Could you check a few things on this model? Use its own coordinates, in mm. Round coordinates to 2 decimals unless told otherwise and drop trailing zeros. Loops run counter-clockwise (first coordinate to the right, second up) from the corner with the lowest first, then second, coordinate; pieces in that order, holes last. Notation, with made-up numbers: M 89.5,19.5 L 146.5,19.5 A12 cw 146.5,39.5 Z; hole C -27,24.5 d6. An arc over 180 degrees is marked long. Answer in a Markdown table with one row per item.
```python
from build123d import *

# Parameters (mm, degrees)
SKETCH1_R           = 1.65
SKETCH1_R_2         = 2.7
BOSS_EXTRUDE1_DEPTH = 6.35


with BuildPart() as part:
    # Sketch1 → Boss-Extrude1 (new body)
    with BuildSketch(Plane(origin=(-388.62, 0, 0), x_dir=(0, -1, 0), z_dir=(-1, 0, 0))):
        Polygon((-371.45, -148.811863322), (-365.1, -148.811863322), (-365.1, -186.911863322), (-328.298226018, -196.772868941), (-329.941726955, -202.906497938), (-305.407210967, -209.480501683), (-303.763710031, -203.346872686), (-194.817257994, -232.538986528), (-196.46075893, -238.672615525), (-171.926242943, -245.24661927), (-170.282742006, -239.112990273), (-61.336289969, -268.305104115), (-62.979790906, -274.438733112), (-38.445274918, -281.012736857), (-36.801773982, -274.87910786), (0, -284.740113479), (0, -3.788281448), (-365.1, -3.788281448), (-365.1, -41.888281448), (-371.45, -41.888281448), (-371.45, -67.288281448), (-365.1, -67.288281448), (-365.1, -123.411863322), (-371.45, -123.411863322), align=None)
        with Locations(Location((-49.890782444, -274.658920486, 0), (0, 0, 90))):
            Circle(SKETCH1_R, mode=Mode.SUBTRACT)
        with Locations(Location((-368.275, -54.588281448, 0), (0, 0, 90))):
            Circle(SKETCH1_R, mode=Mode.SUBTRACT)
        with Locations(Location((-183.371750468, -238.892802899, 0), (0, 0, 90))):
            Circle(SKETCH1_R, mode=Mode.SUBTRACT)
        with Locations(Location((-368.275, -136.111863322, 0), (0, 0, 90))):
            Circle(SKETCH1_R, mode=Mode.SUBTRACT)
        with Locations(Location((-316.852718493, -203.126685312, 0), (0, 0, 90))):
            Circle(SKETCH1_R, mode=Mode.SUBTRACT)
        with Locations(Location((-294.45, -29.188301448, 0), (0, 0, 90))):
            Circle(SKETCH1_R_2, mode=Mode.SUBTRACT)
        with Locations(Location((-207.55, -29.188301448, 0), (0, 0, 90))):
            Circle(SKETCH1_R_2, mode=Mode.SUBTRACT)
        with Locations(Location((-120.65, -29.188301448, 0), (0, 0, 90))):
            Circle(SKETCH1_R_2, mode=Mode.SUBTRACT)
        with Locations(Location((-33.74898, -181.588301448, 0), (0, 0, 90))):
            Circle(SKETCH1_R_2, mode=Mode.SUBTRACT)
        with Locations(Location((-33.74898, -29.188301448, 0), (0, 0, 90))):
            Circle(SKETCH1_R_2, mode=Mode.SUBTRACT)
        with Locations(Location((-33.74898, -130.788301448, 0), (0, 0, 90))):
            Circle(SKETCH1_R_2, mode=Mode.SUBTRACT)
        with Locations(Location((-33.74898, -79.988301448, 0), (0, 0, 90))):
            Circle(SKETCH1_R_2, mode=Mode.SUBTRACT)
    extrude(amount=-BOSS_EXTRUDE1_DEPTH)


solid = part.part
```
1) I want a section at A-A, the plane z = -158. Please give me the cut outline in (x, y), plus the area to 3 significant figures.
Computed:
| item | result |
|---|---|
| outline | M -388.62,0 L -382.27,0 L -382.27,365.1 L -388.62,365.1 Z |
| area | 2,320 mm² |
2) I want a section at B-B, the plane y = 272. Please give me the cut outline in (x, z), plus the area to 3 significant figures.
Computed:
| item | result |
|---|---|
| outline | M -388.62,-211.86 L -382.27,-211.86 L -382.27,-3.79 L -388.62,-3.79 Z |
| area | 1,320 mm² |
3) Will these pins go through, and if not, where does the flat tip stop? P1, Ø3, axis at x = -384, z = -24.5, coming from the +Y side; P2, Ø4.5, axis at y = 33.75, z = -181.59, coming from the +X side; P3, Ø1.9, axis at x = -385.5, y = 367.5, coming from the +Z side; P4, Ø1.9, axis at x = -385, y = 367.5, coming from the -Z side.
Computed:
| item | result |
|---|---|
| P1 | stops at y = 365.1 |
| P2 | passes through |
| P3 | stops at z = -41.89 |
| P4 | stops at z = -148.81 |
4) I need wall thicknesses on line 1 (Y direction, x = -385, z = -29.5); line 2 (Y direction, x = -383, z = -55); line 3 (Y direction, x = -385.5, z = -136). Which ranges of each line are inside material? Lowest first, please.
Computed:
| item | result |
|---|---|
| line 1 | y = 0 to 31.07, 36.43 to 117.97, 123.33 to 204.87, 210.23 to 291.77, 297.13 to 365.1 |
| line 2 | y = 0 to 366.68, 369.87 to 371.45 |
| line 3 | y = 0 to 366.63, 369.92 to 371.45 |
5) If we mould it in two halves opening along Y, with no side actions, what happens to faces 1 (the face through (-382.27, 188, -111)), 2 (the face through (-385.489, 346.957, -191.773)), 3 (the face through (-385.49, 18.66, -279.74))? For each: released by +Y, released by -Y, zero draft, split by the parting line, or undercut.
Computed:
| item | result |
|---|---|
| face 1 | zero draft |
| face 2 | released by +Y |
| face 3 | undercut |
